```python
from build123d import *

# Parameters (mm, degrees)
SKETCH3_R           = 2.5
BOSS_EXTRUDE4_DEPTH = 5
SKETCH4_W           = 3
SKETCH4_H           = 240
BOSS_EXTRUDE5_DEPTH = 40
SKETCH7_R           = 3
CUT_EXTRUDE1_DEPTH  = 10
CUT_EXTRUDE2_DEPTH  = 10


with BuildPart() as part:
    # Sketch3 → Boss-Extrude4 (new body)
    with BuildSketch(Plane(origin=(0, 0, 0), x_dir=(1, 0, 0), z_dir=(0, 1, 0))):
        with BuildLine():
            Line((161.369142032, 10), (170, 10))
            ThreePointArc((170, 10), (180, 0), (170, -10))
            Line((170, -10), (161.369142032, -10))
            ThreePointArc((161.369142032, -10), (152.849946816, -13.180462695), (148.499210458, -21.165644172))
            ThreePointArc((148.499210458, -21.165644172), (106.066017178, -106.066017178), (21.165644172, -148.499210458))
            ThreePointArc((21.165644172, -148.499210458), (13.180462695, -152.849946816), (10, -161.369142032))
            Line((10, -161.369142032), (10, -170))
            ThreePointArc((10, -170), (0, -180), (-10, -170))
            Line((-10, -170), (-10, -161.369142032))
            ThreePointArc((-10, -161.369142032), (-13.180462695, -152.849946816), (-21.165644172, -148.499210458))
            ThreePointArc((-21.165644172, -148.499210458), (-106.066017178, -106.066017178), (-148.499210458, -21.165644172))
            ThreePointArc((-148.499210458, -21.165644172), (-152.849946816, -13.180462695), (-161.369142032, -10))
            Line((-161.369142032, -10), (-170, -10))
            ThreePointArc((-170, -10), (-180, 0), (-170, 10))
            Line((-170, 10), (-161.369142032, 10))
            ThreePointArc((-161.369142032, 10), (-152.849946816, 13.180462695), (-148.499210458, 21.165644172))
            ThreePointArc((-148.499210458, 21.165644172), (-106.066017178, 106.066017178), (-21.165644172, 148.499210458))
            ThreePointArc((-21.165644172, 148.499210458), (-13.180462695, 152.849946816), (-10, 161.369142032))
            Line((-10, 161.369142032), (-10, 170))
            ThreePointArc((-10, 170), (0, 180), (10, 170))
            Line((10, 170), (10, 161.369142032))
            ThreePointArc((10, 161.369142032), (13.180462695, 152.849946816), (21.165644172, 148.499210458))
            ThreePointArc((21.165644172, 148.499210458), (106.066017178, 106.066017178), (148.499210458, 21.165644172))
            ThreePointArc((148.499210458, 21.165644172), (152.849946816, 13.180462695), (161.369142032, 10))
        make_face()
        with Locations((0, 170)):
            Circle(SKETCH3_R, mode=Mode.SUBTRACT)
        with Locations((170, 0)):
            Circle(SKETCH3_R, mode=Mode.SUBTRACT)
        with Locations((0, -170)):
            Circle(SKETCH3_R, mode=Mode.SUBTRACT)
        with Locations((-170, 0)):
            Circle(SKETCH3_R, mode=Mode.SUBTRACT)
    extrude(amount=-BOSS_EXTRUDE4_DEPTH)

    # Sketch4 → Boss-Extrude5 (add)
    with BuildSketch(Plane.XZ.offset(5)):
        Rectangle(SKETCH4_W, SKETCH4_H)
        with Locations((10.5, 0)):
            Rectangle(SKETCH4_W, SKETCH4_H)
        with Locations((21, 0)):
            Rectangle(SKETCH4_W, SKETCH4_H)
        with Locations((31.5, 0)):
            Rectangle(SKETCH4_W, SKETCH4_H)
        with Locations((42, 0)):
            Rectangle(SKETCH4_W, SKETCH4_H)
        with Locations((52.5, 0)):
            Rectangle(SKETCH4_W, SKETCH4_H)
        with Locations((63, 0)):
            Rectangle(SKETCH4_W, SKETCH4_H)
        with Locations((73.5, 0)):
            Rectangle(SKETCH4_W, SKETCH4_H)
        with Locations((84, 0)):
            Rectangle(SKETCH4_W, SKETCH4_H)
        with Locations((-84, 0)):
            Rectangle(SKETCH4_W, SKETCH4_H)
        with Locations((-73.5, 0)):
            Rectangle(SKETCH4_W, SKETCH4_H)
        with Locations((-63, 0)):
            Rectangle(SKETCH4_W, SKETCH4_H)
        with Locations((-52.5, 0)):
            Rectangle(SKETCH4_W, SKETCH4_H)
        with Locations((-42, 0)):
            Rectangle(SKETCH4_W, SKETCH4_H)
        with Locations((-31.5, 0)):
            Rectangle(SKETCH4_W, SKETCH4_H)
        with Locations((-21, 0)):
            Rectangle(SKETCH4_W, SKETCH4_H)
        with Locations((-10.5, 0)):
            Rectangle(SKETCH4_W, SKETCH4_H)
    extrude(amount=BOSS_EXTRUDE5_DEPTH)

    # Sketch7 → Cut-Extrude1 (cut)
    with BuildSketch(Plane(origin=(0, 0, 0), x_dir=(1, 0, 0), z_dir=(0, 1, 0))):
        with Locations((-127.088241501, 0)):
            Circle(SKETCH7_R)
        with Locations((0, 140.377871213)):
            Circle(SKETCH7_R)
        with Locations((0, -140.377871213)):
            Circle(SKETCH7_R)
        with Locations((127.088241501, 0)):
            Circle(SKETCH7_R)
    extrude(amount=-CUT_EXTRUDE1_DEPTH, mode=Mode.SUBTRACT)

    # Sketch8 → Cut-Extrude2 (cut)
    with BuildSketch(Plane(origin=(0, 0, 0), x_dir=(1, 0, 0), z_dir=(0, 1, 0))):
        with BuildLine():
            ThreePointArc((24.849797215, -147.927305047), (40.464884917, -144.438890499), (55.619572151, -139.307082353))
            ThreePointArc((55.619572151, -139.307082353), (36.148630526, -129.032075513), (24.849797215, -147.927305047))
        make_face()
        with BuildLine():
            ThreePointArc((-55.619572151, -139.307082353), (-36.148630526, -129.032075513), (-24.849797215, -147.927305047))
            ThreePointArc((-24.849797215, -147.927305047), (-40.464884917, -144.438890499), (-55.619572151, -139.307082353))
        make_face()
        with BuildLine():
            ThreePointArc((-139.307082353, -55.619572151), (-129.032075513, -36.148630526), (-147.927305047, -24.849797215))
            ThreePointArc((-147.927305047, -24.849797215), (-144.438890499, -40.464884917), (-139.307082353, -55.619572151))
        make_face()
        with BuildLine():
            ThreePointArc((-139.307082353, 55.619572151), (-129.032075513, 36.148630526), (-147.927305047, 24.849797215))
            ThreePointArc((-147.927305047, 24.849797215), (-144.438890499, 40.464884917), (-139.307082353, 55.619572151))
        make_face()
        with BuildLine():
            ThreePointArc((-55.619572151, 139.307082353), (-36.148630526, 129.032075513), (-24.849797215, 147.927305047))
            ThreePointArc((-24.849797215, 147.927305047), (-40.464884917, 144.438890499), (-55.619572151, 139.307082353))
        make_face()
        with BuildLine():
            ThreePointArc((55.619572151, 139.307082353), (36.148630526, 129.032075513), (24.849797215, 147.927305047))
            ThreePointArc((24.849797215, 147.927305047), (40.464884917, 144.438890499), (55.619572151, 139.307082353))
        make_face()
        with BuildLine():
            ThreePointArc((139.307082353, 55.619572151), (129.032075513, 36.148630526), (147.927305047, 24.849797215))
            ThreePointArc((147.927305047, 24.849797215), (144.438890499, 40.464884917), (139.307082353, 55.619572151))
        make_face()
        with BuildLine():
            ThreePointArc((139.307082353, -55.619572151), (129.032075513, -36.148630526), (147.927305047, -24.849797215))
            ThreePointArc((147.927305047, -24.849797215), (144.438890499, -40.464884917), (139.307082353, -55.619572151))
        make_face()
    extrude(amount=-CUT_EXTRUDE2_DEPTH, mode=Mode.SUBTRACT)


solid = part.part
```
Input: part model. Units: mm. Frame: model coordinates. A direction names the side the tool comes from. Give positions to 0.01 mm unless a question says otherwise; leave off trailing zeros. Order: outer loops, then holes, each group sorted by start corner. A loop starts at its lowest first (then second) coordinate and runs counter-clockwise, first axis right, second up.
1. Material intervals for L1, parallel to Z at x = 0, y = -3; L2, parallel to X at y = -2.7, z = 0; L3, parallel to Y at x = -66.5, z = -125, sorted ascending.
Derived:
L1: z = -180 to -172.5, -167.5 to -143.38, -137.38 to 137.38, 143.38 to 167.5, 172.5 to 180
L2: x = -180 to -172.5, -167.5 to -130.09, -124.09 to 124.09, 130.09 to 167.5, 172.5 to 180
L3: y = -5 to 0
2. Section A-A on y = -37. Give the number of separate pieces and of enclosed holes in the cut face, and give its area (3 significant figures).
Derived:
separate pieces: 17
enclosed holes: 0
area: 12,200 mm2
3. Pin query (flat end, axial travel): pin 1 (12 mm diameter, centred on y = -25.5, z = -58.5, fed in from -X); pin 2 (2.5 mm diameter, centred on y = -3.5, z = -165, fed in from +X); pin 3 (2.5 mm diameter, centred on x = 52, y = -25.5, fed in from +Z). Return the tip coordinate at first contact, or that it passes through.
Derived:
pin 1: stops at x = -85.5
pin 2: stops at x = 10
pin 3: stops at z = 120
4. Section B-B on x = 101. Return the cut outline in (y, z), and give its area (3 significant figures).
Derived:
outline: (-5, -110.9) - (0, -110.9) - (0, 110.9) - (-5, 110.9) - close
area: 1,110 mm2
5. Mould query, pull axis X, two halves, no side actions, for faces 1 (the cylindrical face through (152.75, -2.46, -13.27)), 2 (the flat face through (-72, -25, -2)), 3 (the cylindrical face through (0, -2, -180)). Classes: released by +X, released by -X, zero draft, split by the parting line, or undercut.
Derived:
face 1: released by +X
face 2: undercut
face 3: split by the parting line
6. Reachability of faces 4 (the flat face through (-64.5, -25, -2)), 5 (the flat face through (3, 0, -3)), 6 (the flat face through (-85.5, -25, -2)) from +Z, -Z, +X, -X, +Y, -Y: full face, straight path, thin tool, end or side. Return the list, or none.
Derived:
face 4: +Z, -Z, -Y
face 5: +Z, -Z, +X, -X, +Y
face 6: +Z, -Z, -X, -Y
